Design review of the part built by this model. Coordinates are the model's own, in mm. A direction names the side the tool comes from. Give positions to 0.01 mm unless a question says otherwise; leave off trailing zeros. Order: outer loops, then holes, each group sorted by start corner. A loop starts at its lowest first (then second) coordinate and runs counter-clockwise, first axis right, second up. Notation, with made-up numbers: (34, 69.5) -> (59, 69.5) arc R30 cw to (59, 101.5) -> close; hole circle Ø10 at (19, 89.25). An arc over 180 degrees is marked (long way). Return JSON: item names as keys, results as strings.
```python
from build123d import *

# Parameters (mm, degrees)
SKETCH1_W           = 40
SKETCH1_H           = 104.6
BOSS_EXTRUDE1_DEPTH = 4
SKETCH2_R           = 1.65
CUT_EXTRUDE1_DEPTH  = 57.136351859
SKETCH3_R           = 2.25
CUT_EXTRUDE2_DEPTH  = 57.136351859
SKETCH4_R           = 1.45
SKETCH4_W           = 26
SKETCH4_H           = 24
CUT_EXTRUDE3_DEPTH  = 57.136351859
FILLET1_R           = 1


with BuildPart() as part:
    # Sketch1 → Boss-Extrude1 (new body)
    with BuildSketch(Plane(origin=(0, 0, 0), x_dir=(1, 0, 0), z_dir=(0, 1, 0))):
        Rectangle(SKETCH1_W, SKETCH1_H)
    extrude(amount=BOSS_EXTRUDE1_DEPTH)

    # Sketch2 → Cut-Extrude1 (cut, through all)
    with BuildSketch(Plane(origin=(0, 4, 0), x_dir=(1, 0, 0), z_dir=(0, 1, 0))):
        with Locations(Location((-15, 48.8, 0), (0, 0, 270))):
            Circle(SKETCH2_R)
        with Locations(Location((15, 48.8, 0), (0, 0, 270))):
            Circle(SKETCH2_R)
        with Locations(Location((-15, -12.2, 0), (0, 0, 270))):
            Circle(SKETCH2_R)
        with Locations(Location((15, -12.2, 0), (0, 0, 270))):
            Circle(SKETCH2_R)
    extrude(amount=-CUT_EXTRUDE1_DEPTH, mode=Mode.SUBTRACT)

    # Sketch3 → Cut-Extrude2 (cut, through all)
    with BuildSketch(Plane(origin=(0, 4, 0), x_dir=(1, 0, 0), z_dir=(0, 1, 0))):
        with Locations(Location((-5, 31.71959884, 0), (0, 0, 270))):
            Circle(SKETCH3_R)
        with Locations(Location((5, 31.71959884, 0), (0, 0, 270))):
            Circle(SKETCH3_R)
        with Locations(Location((-5, -15.48040116, 0), (0, 0, 270))):
            Circle(SKETCH3_R)
        with Locations(Location((5, -15.48040116, 0), (0, 0, 270))):
            Circle(SKETCH3_R)
        Polygon((-1.15, 31.21959884), (-1.15, 28.61959884), (-10.4, 28.61959884), (-10.4, -12.38040116), (-1.15, -12.38040116), (-1.15, -14.98040116), (1.15, -14.98040116), (1.15, -12.38040116), (10.4, -12.38040116), (10.4, 28.61959884), (1.15, 28.61959884), (1.15, 31.21959884), align=None)
    extrude(amount=-CUT_EXTRUDE2_DEPTH, mode=Mode.SUBTRACT)

    # Sketch4 → Cut-Extrude3 (cut, through all)
    with BuildSketch(Plane(origin=(0, 4, 0), x_dir=(1, 0, 0), z_dir=(0, 1, 0))):
        with Locations(Location((-16.5, -31.3, 0), (0, 0, 270))):
            Circle(SKETCH4_R)
        with Locations(Location((-16.5, -48.8, 0), (0, 0, 270))):
            Circle(SKETCH4_R)
        with Locations(Location((16.5, -31.3, 0), (0, 0, 270))):
            Circle(SKETCH4_R)
        with Locations(Location((16.5, -48.8, 0), (0, 0, 270))):
            Circle(SKETCH4_R)
        with Locations((0, -40.3)):
            Rectangle(SKETCH4_W, SKETCH4_H)
    extrude(amount=-CUT_EXTRUDE3_DEPTH, mode=Mode.SUBTRACT)

    # Fillet1
    fillet1_edges = [part.edges().sort_by_distance(p)[0] for p in [
        (-13, 2, 52.3),
        (-13, 2, 28.3),
        (13, 2, 28.3),
        (13, 2, 52.3),
        (1.15, 2, 12.38040116),
        (-1.15, 2, 12.38040116),
        (-1.15, 2, -28.61959884),
        (1.15, 2, -28.61959884),
        (20, 2, 52.3),
        (-20, 2, 52.3),
        (-20, 2, -52.3),
        (20, 2, -52.3),
    ]]
    fillet(fillet1_edges, radius=FILLET1_R)


solid = part.part
```
Item 1: Mouldability with a two-part tool opening along Z and no side actions: class faces 1 (the face through (20, 2, 1)), 2 (the face through (6, 2, 12.38)), 3 (the face through (10.4, 2, -8)), 4 (the face through (16, 2, 52.3)) as released by +Z, released by -Z, zero draft, split by the parting line, or undercut.
Result set:
{"face 1": "zero draft", "face 2": "undercut", "face 3": "undercut", "face 4": "released by +Z"}
Item 2: For pin 1 (12 mm diameter, centred on x = -5, z = -28, fed in from -Y); pin 2 (1.8 mm diameter, centred on x = 0, y = 2.5, fed in from +Z), all flat-tipped, find the tip position at first contact; note any pin that passes through.
Result set:
{"pin 1": "stops at y = 0", "pin 2": "stops at z = 28.3"}
Item 3: Add section C-C (z = -15.5). Give the boundary of the cut face in (x, y), plus the area to 3 significant figures.
Result set:
{"outline": "(-20, 0) -> (-10.4, 0) -> (-10.4, 4) -> (-20, 4) -> close; (10.4, 0) -> (20, 0) -> (20, 4) -> (10.4, 4) -> close", "area": "76.8 mm^2"}
Item 4: Add section A-A (z = 48.8). Give the boundary of the cut face in (x, y).
Result set:
{"outline": "(-20, 0) -> (-17.95, 0) -> (-17.95, 4) -> (-20, 4) -> close; (-15.05, 0) -> (-13, 0) -> (-13, 4) -> (-15.05, 4) -> close; (13, 0) -> (15.05, 0) -> (15.05, 4) -> (13, 4) -> close; (17.95, 0) -> (20, 0) -> (20, 4) -> (17.95, 4) -> close"}
Item 5: Add section B-B (x = -9). Give the boundary of the cut face in (y, z).
Result set:
{"outline": "(0, -52.3) -> (4, -52.3) -> (4, -28.62) -> (0, -28.62) -> close; (0, 12.38) -> (4, 12.38) -> (4, 28.3) -> (0, 28.3) -> close"}
Item 6: Wall thickness on L1, parallel to X at y = 1.75, z = 12.2; L2, parallel to X at y = 0.8, z = 31.5; L3, parallel to Z at x = -16, y = 2.4: over which ranges is each line inside the solid? List them lowest first. Write a range as [from, to].
Result set:
{"L1": "x = [-20, -16.65], [-13.35, -10.4], [10.4, 13.35], [16.65, 20]", "L2": "x = [-20, -17.94], [-15.06, -13], [13, 15.06], [17.94, 20]", "L3": "z = [-52.3, -50.11], [-47.49, 10.89], [13.51, 29.94], [32.66, 47.44], [50.16, 52.3]"}
Item 7: Add section D-D (x = 5). Give the boundary of the cut face in (y, z).
Result set:
{"outline": "(0, -52.3) -> (4, -52.3) -> (4, -33.97) -> (0, -33.97) -> close; (0, -29.47) -> (4, -29.47) -> (4, -28.62) -> (0, -28.62) -> close; (0, 12.38) -> (4, 12.38) -> (4, 13.23) -> (0, 13.23) -> close; (0, 17.73) -> (4, 17.73) -> (4, 28.3) -> (0, 28.3) -> close"}
Item 8: Machinability: for faces 5 (the face through (-6, 2, -28.62)), 6 (the face through (-17, 2, 52.3)), 7 (the face through (-13, 2, 40)), which of the approach directions +Z, -Z, +X, -X, +Y, -Y give a long, thin tool a straight path to every point of the face, cutting with its end or side? Answer none if there is none.
Result set:
{"face 5": "+Y, -Y", "face 6": "+Z, +X, -X, +Y, -Y", "face 7": "+Z, +Y, -Y"}
